```python
from build123d import *

# Parameters (mm, degrees)
F1_DEPTH = 76.2
F2_W     = 127.0025914325
F2_H     = 25.4
F3_DEPTH = 25.4
F5_DEPTH = 25.4


with BuildPart() as f1:
    # F0 (on Front) → F1 (new body)
    with BuildSketch(Plane.XZ):
        Polygon((-100.3097782258, 25.4), (-125.7071867934, 25.0371804097), (-125.7071867934, -25.7628195903), (26.6928132066, -25.7628195903), (26.6928132066, 0), (-100.3097782258, 0), align=None)
    extrude(amount=F1_DEPTH)

    # F2 (on face) → F3 (join)
    with BuildSketch(Plane.XY):
        with Locations((-36.8084825096, -38.1)):
            Rectangle(F2_W, F2_H)
    extrude(amount=F3_DEPTH)

    # F4 (on face) → F5 (cut)
    with BuildSketch(Plane.XZ.offset(50.8)):
        Polygon((26.6928132066, 25.4), (-100.3097782258, 25.4), (26.6928132066, 0), align=None)
    extrude(amount=-F5_DEPTH, mode=Mode.SUBTRACT)


solid = f1.part
```
Input: part model. Units: mm. Frame: model coordinates. A direction names the side the tool comes from. Give positions to 0.01 mm unless a question says otherwise; leave off trailing zeros. Order: outer loops, then holes, each group sorted by start corner. A loop starts at its lowest first (then second) coordinate and runs counter-clockwise, first axis right, second up. Notation, with made-up numbers: (68, -15) - (107, -15) arc R11 ccw to (107, -7) - close; hole circle Ø5 at (85, 37). An arc over 180 degrees is marked (long way). One line per item, written item: value.
1. Cut plane B-B, the plane x = -11. Output: boundary loops of the cut face in (y, z), and give its area (3 significant figures).
Determined:
outline: (-76.2, -25.76) - (0, -25.76) - (0, 0) - (-25.4, 0) - (-25.4, 7.54) - (-50.8, 7.54) - (-50.8, 0) - (-76.2, 0) - close
area: 2,150 mm2
2. Cut plane C-C, the plane z = 12.5. Output: boundary loops of the cut face in (x, y), and give its area (3 significant figures).
Determined:
outline: (-125.71, -76.2) - (-100.31, -76.2) - (-100.31, -50.8) - (-35.81, -50.8) - (-35.81, -25.4) - (-100.31, -25.4) - (-100.31, 0) - (-125.71, 0) - close
area: 3,570 mm2
3. Reachability of faces 1 (the face through (-52, -25.4, 10)), 2 (the face through (-100.31, -63, 13)), 3 (the face through (-68, -76.2, -11)) from +Z, -Z, +X, -X, +Y, -Y: full face, straight path, thin tool, end or side. Return the list, or none.
Determined:
face 1: +Z, +X, +Y
face 2: +Z, +X, -Y
face 3: +Z, -Z, +X, -X, -Y
4. Cut plane A-A, the plane y = -40. Output: boundary loops of the cut face in (x, z).
Determined:
outline: (-125.71, -25.76) - (26.69, -25.76) - (26.69, 0) - (-100.31, 25.4) - (-125.71, 25.04) - close
5. Cut plane D-D, the plane y = -57. Output: boundary loops of the cut face in (x, z), and give its area (3 significant figures).
Determined:
outline: (-125.71, -25.76) - (26.69, -25.76) - (26.69, 0) - (-100.31, 0) - (-100.31, 25.4) - (-125.71, 25.04) - close
area: 4,570 mm2
6. Pin query (flat end, axial travel): pin 1 Ø7.5 at (x, y) = (-51, -6.5) entering from +Z; pin 2 Ø5 at (x, y) = (-54, -51.5) entering from +Z; pin 3 Ø12.5 at (y, z) = (-65, 9) entering from +X. Return the tip coordinate at first contact, or that it passes through.
Determined:
pin 1: z = 0
pin 2: z = 16.62
pin 3: x = -100.31
7. Line query: probe 1 along Y at (x, z) = (-56.5, 0.5); probe 2 along Z at (x, y) = (-89, -18); probe 3 along X at (y, z) = (-58, 14.5). Output: solid intervals per line, ascending.
Determined:
probe 1: -50.8 to -25.4
probe 2: -25.76 to 0
probe 3: -125.71 to -100.31
